Could you check a few things on this model? Use its own coordinates, in mm. A direction names the side the tool comes from. Give positions to 0.01 mm unless a question says otherwise; leave off trailing zeros. Order: outer loops, then holes, each group sorted by start corner. A loop starts at its lowest first (then second) coordinate and runs counter-clockwise, first axis right, second up. Notation, with made-up numbers: (61, -5) - (90, -5) arc R19 cw to (90, 27) - close; hole circle Ø4 at (3.25, 6.25). An arc over 180 degrees is marked (long way). Put each result on its own line as item: value.
from build123d import *

# Parameters (mm, degrees)
BOSS_EXTRUDE1_DEPTH     = 15
BOSS_EXTRUDE2_DEPTH     = 3
BOSS_EXTRUDE3_DEPTH     = 15
CUT_EXTRUDE1_DEPTH      = 45.988887517
FILLET2_R               = 2
BOSS_EXTRUDE4_DEPTH     = 18
SKETCH8_R               = 2.2
CUT_EXTRUDE3_DEPTH      = 6
FILLET3_R               = 5
FILLET4_SIZE            = 2
CUT_EXTRUDE4_DEPTH      = 51.039984013
CUT_EXTRUDE4_DEPTH_BACK = 51.039984013
SKETCH9_R               = 2.1
SKETCH10_R              = 3.85
CUT_EXTRUDE5_DEPTH      = 8


with BuildPart() as part:
    # Sketch1 → Boss-Extrude1 (new body)
    with BuildSketch(Plane.XY):
        Polygon((0, 0), (30, 0), (30, -8), (2.911761874, -8), align=None)
    extrude(amount=BOSS_EXTRUDE1_DEPTH)

    # Sketch2 → Boss-Extrude2 (add)
    with BuildSketch(Plane.XY.offset(15)):
        Polygon((-11.425184054, 8), (-2.689898432, -16), (38, -16), (38, 8), align=None)
    extrude(amount=BOSS_EXTRUDE2_DEPTH)

    # Sketch3 → Boss-Extrude3 (add)
    with BuildSketch(Plane(origin=(0, 0, 0), x_dir=(-1, 0, 0), z_dir=(0, 0, -1))):
        Polygon((5.712592027, 4), (-34, 4), (-34, -12), (-34, -16), (-38, -16), (-38, 8), (11.425184054, 8), (2.689898432, -16), (-1.566812658, -16), (-0.110931721, -12), align=None)
    extrude(amount=-BOSS_EXTRUDE3_DEPTH)

    # Sketch4 → Cut-Extrude1 (cut, through all)
    with BuildSketch(Plane(origin=(0, 0, 0), x_dir=(-1, 0, 0), z_dir=(0, 0, -1))):
        Polygon((-38, 8), (-34, 8), (-34, -12), (4.145779369, -12), (4.145779369, -16), (-30, -16), (-38, -16), align=None)
    extrude(amount=-CUT_EXTRUDE1_DEPTH, mode=Mode.SUBTRACT)

    # Fillet2
    fillet2_edges = [part.edges().sort_by_distance(p)[0] for p in [
        (-5.712592027, 4, 7.5),
    ]]
    fillet(fillet2_edges, radius=FILLET2_R)

    # Sketch5 → Boss-Extrude4 (add)
    with BuildSketch(Plane(origin=(0, 0, 0), x_dir=(-1, 0, 0), z_dir=(0, 0, -1))):
        Polygon((11.425184054, 8), (20.160469676, 32), (-34, 32), (-34, 8), align=None)
    extrude(amount=-BOSS_EXTRUDE4_DEPTH)

    # Sketch7 → Cut-Revolve1 (revolve, cut)
    with BuildSketch(Plane(origin=(0, 0, 0), x_dir=(-1, 0, 0), z_dir=(0, 0, -1))):
        Polygon((-34, 17), (14.700916162, 17), (15.883819424, 20.25), (-15, 20.25), (-15, 22.25), (-26.5, 22.25), (-26.5, 28.25), (-34, 28.25), align=None)
    revolve(axis=Axis((34, 17, 0), (-1, 0, 0)), mode=Mode.SUBTRACT)

    # Sketch8 → Cut-Extrude3 (cut)
    with BuildSketch(Plane(origin=(26.5, 0, 0), x_dir=(0, 0, -1), z_dir=(1, 0, 0))):
        with Locations((-5.656854249, 22.656854249)):
            Circle(SKETCH8_R)
        with Locations((5.656854249, 22.656854249)):
            Circle(SKETCH8_R)
        with Locations((5.656854249, 11.343145751)):
            Circle(SKETCH8_R)
        with Locations((-5.656854249, 11.343145751)):
            Circle(SKETCH8_R)
    extrude(amount=-CUT_EXTRUDE3_DEPTH, mode=Mode.SUBTRACT)

    # Fillet3
    fillet3_edges = [part.edges().sort_by_distance(p)[0] for p in [
        (-20.160469676, 32, 9),
    ]]
    fillet(fillet3_edges, radius=FILLET3_R)

    # Fillet4
    fillet4_edges = [part.edges().sort_by_distance(p)[0] for p in [
        (10.490135179, 32, 18),
        (-10.931986058, 6.644949642, 18),
        (-17.115489864, 29.867882182, 18),
        (34, 10, 18),
        (14.927110316, -12, 18),
    ]]
    chamfer(fillet4_edges, length=FILLET4_SIZE)

    # Sketch9 → Cut-Extrude4 (cut, two sides: drawn at the far end of the back side and taken through both)
    with BuildSketch(Plane(origin=(0, 0, 0), x_dir=(-1, 0, 0), z_dir=(0, 0, -1)).offset(-CUT_EXTRUDE4_DEPTH_BACK)):
        with Locations((-11.105422856, 9)):
            Circle(SKETCH9_R)
    extrude(amount=CUT_EXTRUDE4_DEPTH + CUT_EXTRUDE4_DEPTH_BACK, mode=Mode.SUBTRACT)

    # Sketch10 → Cut-Extrude5 (cut)
    with BuildSketch(Plane.XY.offset(18)):
        with Locations((11.105422856, 9)):
            Circle(SKETCH10_R)
    extrude(amount=-CUT_EXTRUDE5_DEPTH, mode=Mode.SUBTRACT)


solid = part.part
1) If I drill on line 1 (Y direction, x = 21, z = 13.75); line 2 (Y direction, x = 9, z = 11.5); line 3 (Z direction, x = 29.5, y = -9.5), over which ranges is the centre line in solid material (lowest first)? Write a range as [from, to].
Filled in:
line 1: y = [-8, 0], [4, 32]
line 2: y = [-8, 0], [4, 5.78], [12.22, 32]
line 3: z = [15, 18]
2) Suppose I cut it at B-B, the plane x = 3.5. List the corners of the cut face in (y, z) for me.
Filled in:
outline: (-12, 15) - (-8, 15) - (-8, 0) - (0, 0) - (0, 15) - (4, 15) - (4, 0) - (13.75, 0) arc R3.25 cw to (20.25, 0) - (32, 0) - (32, 16) - (30, 18) - (-10, 18) - (-12, 16) - close
3) I'm going to push flat-ended pins straight in: pin 1 (3.5 mm diameter, centred on y = 15.5, z = 7, fed in from +X); pin 2 (4 mm diameter, centred on y = 18.5, z = 1.5, fed in from +X); pin 3 (6.5 mm diameter, centred on y = -5, z = 11, fed in from +X). Where does each tip first touch, or does it pass through?
Filled in:
pin 1: stops at x = 26.5
pin 2: stops at x = 15
pin 3: stops at x = 30
4) Suppose I cut it at A-A, the plane z = 4.25. State how many separate pieces and enclosed holes the cut face has, and give its area (3 significant figures).
Filled in:
separate pieces: 2
enclosed holes: 1
area: 1,380 mm^2
5) Suppose I cut it at D-D, the plane x = 22. List the corners of the cut face in (y, z) for me, and give its area (3 significant figures).
Filled in:
outline: (-12, 15) - (-8, 15) - (-8, 0) - (0, 0) - (0, 15) - (4, 15) - (4, 0) - (11.75, 0) arc R5.25 cw to (22.25, 0) - (32, 0) - (32, 16) - (30, 18) - (-10, 18) - (-12, 16) - close; hole circle Ø4.4 at (11.34, 5.66); hole circle Ø4.4 at (22.66, 5.66)
area: 594 mm^2
6) We'd pull the mould along X, two halves only. Please class faces 1 (the flat face through (15, 17, 4)), 2 (the cylindrical face through (9.102, 9.631, 5.07)), 3 (the cylindrical face through (23.54, 24.14, 7.28)), 4 (the cylindrical face through (-17.154, 29.813, 8.112)): pulls with the +X half, pulls with the -X half, needs draft (parallel to the pull), parting line crosses it, or undercut.
Filled in:
face 1: pulls with the +X half
face 2: undercut
face 3: needs draft
face 4: pulls with the -X half
7) Which directions (+Z, -Z, +X, -X, +Y, -Y) give clear straight access to the entire face, cutting with the end or side of a thin tool? Please do faces 5 (the flat face through (13, 7, 10)), 6 (the flat face through (15, 0, 7)), 7 (the flat face through (20.5, 11, 6)).
Filled in:
face 5: +Z
face 6: -Z, +X
face 7: +X
8) Suppose I cut it at C-C, the plane y = 19.5. List the corners of the cut face in (x, z) for me.
Filled in:
outline: (-15.61, 2.08) - (15, 2.08) - (15, 4.62) - (26.5, 4.62) - (26.5, 10.97) - (34, 10.97) - (34, 16) - (32, 18) - (-13.48, 18) - (-15.61, 16) - close
